CAD build for the part. Positions are in the model's coordinates, mm. Face numbers are marked on the shaded views. A direction names the side the tool comes from. Coordinates: 2 decimals unless noted, no trailing zeros. Loops run counter-clockwise (first coordinate to the right, second up) from the corner with the lowest first, then second, coordinate; pieces in that order, holes last. Notation, with made-up numbers: (3.25, -39) -> (54.25, -39) arc R12 cw to (54.25, -16) -> close; hole circle Ø11 at (-37, 71.25). An arc over 180 degrees is marked (long way). Write each question's results on one line, items separated by ' | '.
```python
from build123d import *

# Parameters (mm, degrees)
F0_W       = 31
F0_H       = 8.5
F0_W_2     = 9.5
F0_H_2     = 6.5
F1_DEPTH   = 5
F2_W       = 4
F2_H       = 8.5
F3_DEPTH   = 0.5
F5_DEPTH   = 3.4125
F7_SIZE2   = 0.658252
F7_SIZE    = 4.99999
F7_2_SIZE2 = 0.658252
F7_2_SIZE  = 4.99999
F8_W       = 35
F8_H       = 12.5
F8_W_2     = 31
F8_H_2     = 8.5
F9_DEPTH   = 4
F11_DEPTH  = 4
F12_W      = 15
F12_H      = 5
F13_DEPTH  = 5.5
F14_R      = 1.5875
F15_DEPTH  = 94.6591745177
F16_R      = 2.1


# Not quite as in the source:
# - a fillet or chamfer is up to 0.001 mm smaller than in the source, because OpenCascade refuses the exact size
# - a length typed as a fraction of an inch, garbled in the dataset ("3 / 203.2 mm" for 3/8 in), is restored


with BuildPart() as f1:
    # F0 (on Front) → F1 (new body)
    with BuildSketch(Plane.XZ):
        Polygon((46.25, 17.75), (-57.25, 17.75), (-61.6581745177, -7.25), (50.6581745177, -7.25), align=None)
        Polygon((-48.1899019538, 4.25), (-34.4399019538, 4.25), (-31.6899019538, 1.5), (-31.6899019538, -1.5), (-34.4399019538, -4.25), (-48.1899019538, -4.25), align=None, mode=Mode.SUBTRACT)
        Rectangle(F0_W, F0_H, mode=Mode.SUBTRACT)
        with Locations((32.4399019538, 0)):
            Rectangle(F0_W_2, F0_H_2, mode=Mode.SUBTRACT)
    extrude(amount=-F1_DEPTH)

    # F2 (on face) → F3 (cut)
    with BuildSketch(Plane.XZ):
        with Locations((-17.5, 0)):
            Rectangle(F2_W, F2_H)
    extrude(amount=-F3_DEPTH, mode=Mode.SUBTRACT)

    # F4 (on face) → F5 (cut)
    with BuildSketch(Plane(origin=(0, 5, 0), x_dir=(-1, 0, 0), z_dir=(0, 1, 0))):
        Polygon((-22.1211519538, -5.3578125), (-22.1211519538, 5.3578125), (-42.7586519538, 5.3578125), (-42.7586519538, -5.3578125), align=None)
    extrude(amount=-F5_DEPTH, mode=Mode.SUBTRACT)

    # F7 (size 5 and 0.6582624879 in the source; OpenCascade refuses exactly that, so slightly less here)
    f7_edges = [f1.edges().sort_by_distance(p)[0] for p in [
        (-59.454087, 5, 5.25),
    ]]
    f7_side = f1.faces().sort_by_distance((-59.454087, 2.5, 5.25))[0]
    chamfer(f7_edges, length=F7_SIZE, length2=F7_SIZE2, reference=f7_side)

    # F7#2 (size 5 and 0.6582624879 in the source; OpenCascade refuses exactly that, so slightly less here)
    f7_2_edges = [f1.edges().sort_by_distance(p)[0] for p in [
        (48.454087, 5, 5.25),
    ]]
    f7_2_side = f1.faces().sort_by_distance((48.454087, 2.5, 5.25))[0]
    chamfer(f7_2_edges, length=F7_2_SIZE, length2=F7_2_SIZE2, reference=f7_2_side)

    # F8 (on face) → F9 (join)
    with BuildSketch(Plane(origin=(0, 5, 0), x_dir=(-1, 0, 0), z_dir=(0, 1, 0))):
        Rectangle(F8_W, F8_H)
        Rectangle(F8_W_2, F8_H_2, mode=Mode.SUBTRACT)
    extrude(amount=F9_DEPTH)

    # F10 (on face) → F11 (join)
    with BuildSketch(Plane(origin=(0, 5, 0), x_dir=(-1, 0, 0), z_dir=(0, 1, 0))):
        Polygon((50.1899019538, 6.25), (33.611474829, 6.25), (29.6899019538, 2.3284271247), (29.6899019538, -2.3284271247), (33.611474829, -6.25), (50.1899019538, -6.25), align=None)
        Polygon((31.6899019538, 1.5), (34.4399019538, 4.25), (48.1899019538, 4.25), (48.1899019538, -4.25), (34.4399019538, -4.25), (31.6899019538, -1.5), align=None, mode=Mode.SUBTRACT)
    extrude(amount=F11_DEPTH)

    # F12 (on face) → F13 (join)
    with BuildSketch(Plane.XY.offset(17.75)):
        with Locations((-36.5, 2.5)):
            Rectangle(F12_W, F12_H)
        with Locations((25.5, 2.5)):
            Rectangle(F12_W, F12_H)
        with Locations((-5.5, 2.5)):
            Rectangle(F12_W, F12_H)
    extrude(amount=F13_DEPTH)

    # F14 (on face) → F15 (cut, through all)
    with BuildSketch(Plane.YZ.offset(33)):
        with Locations((2.5, 20.75)):
            Circle(F14_R)
    extrude(amount=-F15_DEPTH, mode=Mode.SUBTRACT)

    # F16
    f16_edges = [f1.edges().sort_by_distance(p)[0] for p in [
        (-36.5, 0, 23.25),
        (-5.5, 0, 23.25),
        (25.5, 0, 23.25),
    ]]
    fillet(f16_edges, radius=F16_R)


solid = f1.part
```
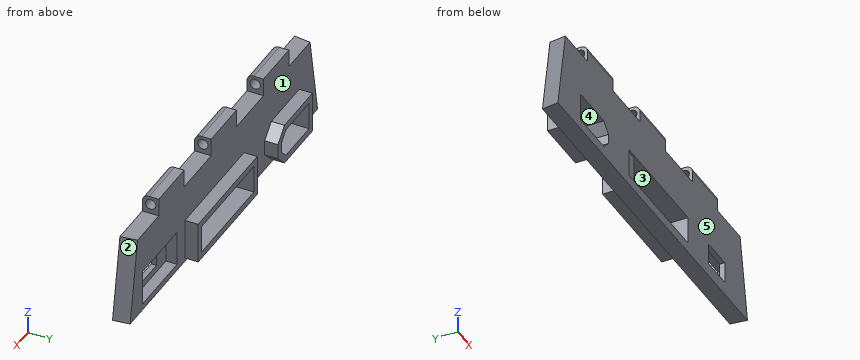
Q1. Drop flat-ended pins along their axis: pin 1 (1 mm diameter, centred on x = 3.5, y = 4.5, fed in from +Z); pin 2 (4 mm diameter, centred on y = 3.5, z = 20, fed in from -X); pin 3 (1.2 mm diameter, centred on x = 6, y = 6.5, fed in from -Z); pin 4 (12 mm diameter, centred on x = -18, z = -1, fed in from -Y). Give the stop position or say it passes through.
Results are:
pin 1: z = 17.75 | pin 2: x = -44 | pin 3: z = -6.25 | pin 4: y = 0
Q2. Pull direction Z, two halves, no side cores. Call the marked faces 1, 2 and 3: +Z half, -Z half, draft (parallel to the pull), parting line (faces both ways), or undercut.
Results are:
face 1: draft | face 2: +Z half | face 3: undercut
Q3. Cut at B-B on y = 6.5. Write the cut outline in (x, z).
Results are:
outline: (-50.19, -6.25) -> (-33.61, -6.25) -> (-29.69, -2.33) -> (-29.69, 2.33) -> (-33.61, 6.25) -> (-50.19, 6.25) -> close; (-17.5, -6.25) -> (17.5, -6.25) -> (17.5, 6.25) -> (-17.5, 6.25) -> close; hole (-48.19, -4.25) -> (-34.44, -4.25) -> (-31.69, -1.5) -> (-31.69, 1.5) -> (-34.44, 4.25) -> (-48.19, 4.25) -> close; hole (-15.5, -4.25) -> (15.5, -4.25) -> (15.5, 4.25) -> (-15.5, 4.25) -> close
Q4. Wall check: L1, parallel to Z at x = -32.5, y = 2.5; L2, parallel to X at y = 5.5, z = 1; L3, parallel to Z at x = 22.75, y = 2.5. Give the ranges that are in metal, low to high. Write a range as from..to.
Results are:
L1: -7.25..-2.31, 2.31..19.16, 22.34..23.25 | L2: -50.19..-48.19, -31.69..-29.69, -17.5..-15.5, 15.5..17.5 | L3: -7.25..-5.36, 5.36..19.16, 22.34..23.25
Q5. Cut at A-A on x = -37.5. Give the number of separate pieces and of enclosed holes in the cut face, and give its area (3 significant figures).
Results are:
separate pieces: 2 | enclosed holes: 1 | area: 117 mm^2
Q6. Cut at C-C on x = 41.5. Write the cut outline in (y, z).
Results are:
outline: (0, -7.25) -> (5, -7.25) -> (5, -5.36) -> (1.59, -5.36) -> (1.59, 5.36) -> (5, 5.36) -> (5, 17.75) -> (0, 17.75) -> close
Q7. Which spindle directions (+Z, -Z, +X, -X, +Y, -Y) get a long thin tool onto all of the face, cutting with end or side? Do the marked faces 4 and 5. Say none if no direction does.
Results are:
face 4: +Y, -Y | face 5: +Z, -Z, +X, -X, -Y
